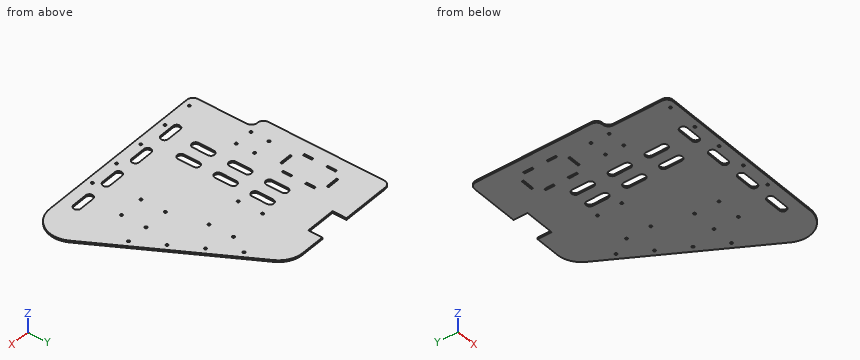
from build123d import *

# Parameters (mm, degrees)
EXTRUDE_1_DEPTH        = 3
SKETCH_2_R             = 2
CUT_EXTRUDE_1_DEPTH    = 10
SKETCH_3_W             = 45
SKETCH_3_H             = 100
CUT_EXTRUDE_2_DEPTH    = 489.651064791
FILLET_1_R             = 10
SKETCH_5_W             = 3
SKETCH_5_H             = 15
SKETCH_5_W_2           = 20
SKETCH_5_H_2           = 3
CUT_EXTRUDE_2593_DEPTH = 10
CUT_EXTRUDE_3695_DEPTH = 10
SKETCH_7_R             = 2
CUT_EXTRUDE_5_DEPTH    = 10


with BuildPart() as part:
    # 草图1 → 凸台-拉伸1 (new body)
    with BuildSketch(Plane.XY):
        with BuildLine():
            Line((0, 66), (0, 0))
            Line((0, 0), (337.717967697, 0))
            ThreePointArc((337.717967697, 0), (372.358983849, 20), (372.358983849, 60))
            Line((372.358983849, 60), (239.568421935, 290))
            ThreePointArc((239.568421935, 290), (224.927405784, 304.641016151), (204.927405784, 310))
            Line((204.927405784, 310), (164.927405784, 310))
            Line((164.927405784, 310), (164.927405784, 287))
            Line((164.927405784, 287), (114.927405784, 287))
            Line((114.927405784, 287), (114.927405784, 310))
            Line((114.927405784, 310), (25, 310))
            Line((25, 310), (25, 66))
            Line((25, 66), (0, 66))
        make_face()
    extrude(amount=EXTRUDE_1_DEPTH)

    # 草图2 → 切除-拉伸1 (cut)
    with BuildSketch(Plane.XY.offset(3)):
        with Locations((262.5, 10)):
            Circle(SKETCH_2_R)
        with Locations((212.5, 10)):
            Circle(SKETCH_2_R)
        with Locations((162.5, 10)):
            Circle(SKETCH_2_R)
        with Locations((112.5, 10)):
            Circle(SKETCH_2_R)
        with Locations((62.5, 10)):
            Circle(SKETCH_2_R)
        with Locations((251.089745962, 250.044481415)):
            Circle(SKETCH_2_R)
        with Locations((276.089745962, 206.743211225)):
            Circle(SKETCH_2_R)
        with Locations((301.089745962, 163.441941036)):
            Circle(SKETCH_2_R)
        with Locations((326.089745962, 120.140670847)):
            Circle(SKETCH_2_R)
    extrude(amount=-CUT_EXTRUDE_1_DEPTH, mode=Mode.SUBTRACT)

    # 草图3 → 切除-拉伸2 (cut, through all)
    with BuildSketch(Plane.XY.offset(3)):
        with Locations((22.5, 50)):
            Rectangle(SKETCH_3_W, SKETCH_3_H)
    extrude(amount=-CUT_EXTRUDE_2_DEPTH, mode=Mode.SUBTRACT)

    # 圆角1
    fillet_1_edges = [part.edges().sort_by_distance(p)[0] for p in [
        (25, 310, 1.5),
        (25, 100, 1.5),
        (45, 100, 1.5),
        (45, 0, 1.5),
    ]]
    fillet(fillet_1_edges, radius=FILLET_1_R - 0.0001)  # a hair under: the kernel refuses the full size

    # 草图5 → Cut-Extrude 2593 (cut)
    with BuildSketch(Plane(origin=(0, 0, 0), x_dir=(-1, 0, 0), z_dir=(0, 0, -1))):
        with Locations((-92, 232.5)):
            Rectangle(SKETCH_5_W, SKETCH_5_H)
        with Locations((-92, 194)):
            Rectangle(SKETCH_5_W, SKETCH_5_H)
        with Locations((-48.5, 194)):
            Rectangle(SKETCH_5_W, SKETCH_5_H)
        with Locations((-48.5, 232.5)):
            Rectangle(SKETCH_5_W, SKETCH_5_H)
        with Locations((-70.25, 251.5)):
            Rectangle(SKETCH_5_W_2, SKETCH_5_H_2)
        with Locations((-70.25, 175)):
            Rectangle(SKETCH_5_W_2, SKETCH_5_H_2)
    extrude(amount=-CUT_EXTRUDE_2593_DEPTH, mode=Mode.SUBTRACT)

    # 草图6 → Cut-Extrude 3695 (cut)
    with BuildSketch(Plane(origin=(0, 0, 0), x_dir=(-1, 0, 0), z_dir=(0, 0, -1))):
        with BuildLine():
            Line((-312.5, 31), (-287.5, 31))
            ThreePointArc((-287.5, 31), (-281.5, 25), (-287.5, 19))
            Line((-287.5, 19), (-312.5, 19))
            ThreePointArc((-312.5, 19), (-318.5, 25), (-312.5, 31))
        make_face()
        with BuildLine():
            Line((-252.5, 19), (-227.5, 19))
            ThreePointArc((-227.5, 19), (-221.5, 25), (-227.5, 31))
            Line((-227.5, 31), (-252.5, 31))
            ThreePointArc((-252.5, 31), (-258.5, 25), (-252.5, 19))
        make_face()
        with BuildLine():
            Line((-192.5, 19), (-167.5, 19))
            ThreePointArc((-167.5, 19), (-161.5, 25), (-167.5, 31))
            Line((-167.5, 31), (-192.5, 31))
            ThreePointArc((-192.5, 31), (-198.5, 25), (-192.5, 19))
        make_face()
        with BuildLine():
            Line((-132.5, 19), (-107.5, 19))
            ThreePointArc((-107.5, 19), (-101.5, 25), (-107.5, 31))
            Line((-107.5, 31), (-132.5, 31))
            ThreePointArc((-132.5, 31), (-138.5, 25), (-132.5, 19))
        make_face()
        with BuildLine():
            Line((-114, 212.5), (-114, 187.5))
            ThreePointArc((-114, 187.5), (-120, 181.5), (-126, 187.5))
            Line((-126, 187.5), (-126, 212.5))
            ThreePointArc((-126, 212.5), (-120, 218.5), (-114, 212.5))
        make_face()
        with BuildLine():
            Line((-144, 212.5), (-144, 187.5))
            ThreePointArc((-144, 187.5), (-150, 181.5), (-156, 187.5))
            Line((-156, 187.5), (-156, 212.5))
            ThreePointArc((-156, 212.5), (-150, 218.5), (-144, 212.5))
        make_face()
        with BuildLine():
            Line((-144, 151.861710405), (-144, 126.861710405))
            ThreePointArc((-144, 126.861710405), (-150, 120.861710405), (-156, 126.861710405))
            Line((-156, 126.861710405), (-156, 151.861710405))
            ThreePointArc((-156, 151.861710405), (-150, 157.861710405), (-144, 151.861710405))
        make_face()
        with BuildLine():
            Line((-144, 91.22342081), (-144, 66.22342081))
            ThreePointArc((-144, 66.22342081), (-150, 60.22342081), (-156, 66.22342081))
            Line((-156, 66.22342081), (-156, 91.22342081))
            ThreePointArc((-156, 91.22342081), (-150, 97.22342081), (-144, 91.22342081))
        make_face()
        with BuildLine():
            Line((-114, 151.861710405), (-114, 126.861710405))
            ThreePointArc((-114, 126.861710405), (-120, 120.861710405), (-126, 126.861710405))
            Line((-126, 126.861710405), (-126, 151.861710405))
            ThreePointArc((-126, 151.861710405), (-120, 157.861710405), (-114, 151.861710405))
        make_face()
        with BuildLine():
            Line((-114, 91.22342081), (-114, 66.22342081))
            ThreePointArc((-114, 66.22342081), (-120, 60.22342081), (-126, 66.22342081))
            Line((-126, 66.22342081), (-126, 91.22342081))
            ThreePointArc((-126, 91.22342081), (-120, 97.22342081), (-114, 91.22342081))
        make_face()
    extrude(amount=-CUT_EXTRUDE_3695_DEPTH, mode=Mode.SUBTRACT)

    # 草图7 → 切除-拉伸5 (cut)
    with BuildSketch(Plane(origin=(0, 0, 0), x_dir=(-1, 0, 0), z_dir=(0, 0, -1))):
        with Locations((-290, 120)):
            Circle(SKETCH_7_R)
        with Locations((-250, 120)):
            Circle(SKETCH_7_R)
        with Locations((-290, 80)):
            Circle(SKETCH_7_R)
        with Locations((-250, 80)):
            Circle(SKETCH_7_R)
        with Locations((-85, 135)):
            Circle(SKETCH_7_R)
        with Locations((-55, 135)):
            Circle(SKETCH_7_R)
        with Locations(Location((-55, 105, 0), (0, 0, 180))):
            Circle(SKETCH_7_R)
        with Locations(Location((-85, 105, 0), (0, 0, 180))):
            Circle(SKETCH_7_R)
        with Locations((-235, 220)):
            Circle(SKETCH_7_R)
        with Locations((-235, 180)):
            Circle(SKETCH_7_R)
        with Locations(Location((-175, 180, 0), (0, 0, 180))):
            Circle(SKETCH_7_R)
        with Locations(Location((-175, 220, 0), (0, 0, 180))):
            Circle(SKETCH_7_R)
    extrude(amount=-CUT_EXTRUDE_5_DEPTH, mode=Mode.SUBTRACT)


solid = part.part
Work out the finished part from the listing and answer in its coordinate system (mm). Coordinates: 2 decimals unless noted, no trailing zeros. Order: outer loops, then holes, each group sorted by start corner. A loop starts at its lowest first (then second) coordinate and runs counter-clockwise, first axis right, second up. Notation, with made-up numbers: (-8.5, 20) - (31.5, 20) arc R18 cw to (31.5, 43) - close; hole circle Ø4 at (7, 59). An arc over 180 degrees is marked (long way). Put each result on its own line as item: value. Start each with the question number.
1) Find section A-A (x = 74). Give the vertices of the cut face in (y, z).
2) Find section B-B (y = 235.5). Give the vertices of the cut face in (x, z), plus the area to 3 significant figures.
3) Find section C-C (z = 0.8). State how many separate pieces and enclosed holes the cut face has, plus the area to 3 significant figures.
4) Find section D-D (y = 279). Give the vertices of the cut face in (x, z).
5) Flat-ended cylindrical pins translate along their axes: pin 1 (0.9 mm diameter, centred on y = 81, z = 2, fed in from -X); pin 2 (0.9 mm diameter, centred on y = 81.5, z = 1.5, fed in from +X); pin 3 (2.5 mm diameter, centred on x = 212.5, y = 10, fed in from -Z). Find the tip coordinate at first contact, or state that the pin passes through.
6) Find the intervals of material crossed by line 1 (Y direction, x = 84.5, z = 0.15); line 2 (Y direction, x = 112, z = 1.4); line 3 (Y direction, x = 175, z = 1.7), in increasing order. Write a range as from..to.
Results list:
1. outline: (0, 0) - (173.5, 0) - (173.5, 3) - (0, 3) - close; (176.5, 0) - (250, 0) - (250, 3) - (176.5, 3) - close; (253, 0) - (310, 0) - (310, 3) - (253, 3) - close
2. outline: (25, 0) - (47, 0) - (47, 3) - (25, 3) - close; (50, 0) - (90.5, 0) - (90.5, 3) - (50, 3) - close; (93.5, 0) - (271.03, 0) - (271.03, 3) - (93.5, 3) - close
2. area: 720 mm^2
3. separate pieces: 1
3. enclosed holes: 37
3. area: 81,600 mm^2
4. outline: (25, 0) - (245.92, 0) - (245.92, 3) - (25, 3) - close
5. pin 1: stops at x = 45
5. pin 2: stops at x = 360.21
5. pin 3: passes through
6. line 1: y = 0..103.06, 106.94..133.06, 136.94..310
6. line 2: y = 0..8.06, 11.94..19, 31..310
6. line 3: y = 0..19, 31..178, 182..218, 222..310
